Work out the finished part from the listing and answer in its coordinate system (mm). Give positions to 0.01 mm unless a question says otherwise; leave off trailing zeros. One line per question, with ' | ' between items. Start each with the question number.
1. Section A-A (z = 2.75) is taken. Give the number of separate pieces and of enclosed holes in the cut face, plus the area to 3 significant figures.
2. Each of these flat-tipped pins is pushed along its axis until it touches: pin 1 (1 mm diameter, centred on y = 23, z = 3, fed in from +X); pin 2 (2.5 mm diameter, centred on x = 35, y = 0, fed in from +Z); pin 3 (1.8 mm diameter, centred on x = -30.31, y = 17.5, fed in from +Z). Where does it stop, or does it pass through?
3. Find the intervals of material crossed by line 1 (Y direction, x = 30, z = -0.75); line 2 (X direction, y = -18, z = 4); line 3 (Y direction, x = -22.5, z = -2), in increasing order.
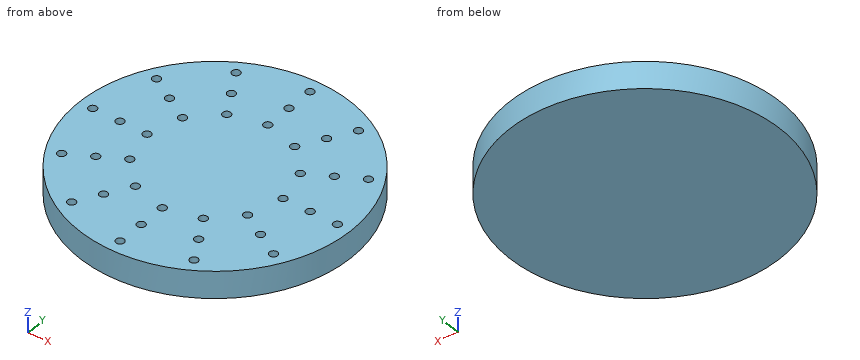
Autodesk Fusion 360 part; units mm, degrees
sketch "base plate" plane through (0, 0, 0) normal (0, 0, 1) x (1, 0, 0)
  circle A0 centre (0, 0) radius 50
  dimension "d1" = 100
extrude "Extrude1" add sketch "base plate" along normal mid plane 10
sketch "tube holes outer layer" plane through (0, 0, 5) normal (0, 0, 1) x (-1, 0, 0)
  circle A0 centre (0, 0) radius 50
  circle A1 centre (45, 0) radius 1.5
  point P0 (-45, 0)
  point P1 (-38.9711, -22.5)
  point P2 (-22.5, -38.9711)
  point P3 (0, -45)
  point P4 (22.5, -38.9711)
  point P5 (38.9711, -22.5)
  point P6 (38.9711, 22.5)
  point P7 (22.5, 38.9711)
  point P8 (0, 45)
  point P9 (-22.5, 38.9711)
  point P10 (-38.9711, 22.5)
  dimension "d4" = 3
  dimension "d6" = 360
hole "Hole1" at (0, 45, 5) at (22.5, 38.9711, 5) at (38.9711, 22.5, 5) at (45, 0, 5) at (38.9711, -22.5, 5) at (22.5, -38.9711, 5) at (0, -45, 5) at (-22.5, -38.9711, 5) at (-38.9711, -22.5, 5) at (-45, 0, 5) at (-38.9711, 22.5, 5) at (-22.5, 38.9711, 5) direction (0, 0, -1) diameter 3 depth 9 tip angle 118
sketch "tube holes layer 2" plane through (0, 0, 5) normal (0, 0, 1) x (-1, 0, 0)
  circle A0 centre (38.9711, -22.5) radius 1.5
  circle A1 centre (38.9711, 22.5) radius 1.5
  circle A2 centre (0, 45) radius 1.5
  circle A3 centre (-38.9711, 22.5) radius 1.5
  circle A4 centre (-38.9711, -22.5) radius 1.5
  circle A5 centre (0, -45) radius 1.5
  circle A6 centre (-22.5, -38.9711) radius 1.5
  circle A7 centre (-45, 0) radius 1.5
  circle A8 centre (-22.5, 38.9711) radius 1.5
  circle A9 centre (22.5, 38.9711) radius 1.5
  circle A10 centre (45, 0) radius 1.5
  circle A11 centre (22.5, -38.9711) radius 1.5
  circle A12 centre (0, 0) radius 50
  line L0 (0, 0) -> (0, -45) construction
  circle A13 centre (0, -35) radius 1.5
  circle A14 centre (0, 35) radius 1.5
  circle A15 centre (-17.5, 30.3109) radius 1.5
  circle A16 centre (-30.3109, 17.5) radius 1.5
  circle A17 centre (-35, 0) radius 1.5
  circle A18 centre (-30.3109, -17.5) radius 1.5
  circle A19 centre (-17.5, -30.3109) radius 1.5
  circle A20 centre (17.5, -30.3109) radius 1.5
  circle A21 centre (30.3109, -17.5) radius 1.5
  circle A22 centre (35, 0) radius 1.5
  circle A23 centre (30.3109, 17.5) radius 1.5
  circle A24 centre (17.5, 30.3109) radius 1.5
  dimension "d10" = 3
  dimension "d12" = 360
hole "Hole2" at (-17.5, 30.3109, 5) at (0, 35, 5) at (17.5, 30.3109, 5) at (30.3109, 17.5, 5) at (35, 0, 5) at (30.3109, -17.5, 5) at (17.5, -30.3109, 5) at (0, -35, 5) at (-17.5, -30.3109, 5) at (-30.3109, -17.5, 5) at (-35, 0, 5) at (-30.3109, 17.5, 5) direction (0, 0, -1) diameter 3 depth 9 tip angle 118
sketch "tube holes layer 3" plane through (0, 0, 5) normal (0, 0, 1) x (-1, 0, 0)
  circle A0 centre (35, 0) radius 1.5
  circle A1 centre (17.5, 30.3109) radius 1.5
  circle A2 centre (-17.5, 30.3109) radius 1.5
  circle A3 centre (-35, 0) radius 1.5
  circle A4 centre (-17.5, -30.3109) radius 1.5
  circle A5 centre (17.5, -30.3109) radius 1.5
  circle A6 centre (0, -35) radius 1.5
  circle A7 centre (-30.3109, -17.5) radius 1.5
  circle A8 centre (-30.3109, 17.5) radius 1.5
  circle A9 centre (0, 35) radius 1.5
  circle A10 centre (30.3109, 17.5) radius 1.5
  circle A11 centre (30.3109, -17.5) radius 1.5
  circle A12 centre (38.9711, -22.5) radius 1.5
  circle A13 centre (38.9711, 22.5) radius 1.5
  circle A14 centre (0, 45) radius 1.5
  circle A15 centre (-38.9711, 22.5) radius 1.5
  circle A16 centre (-38.9711, -22.5) radius 1.5
  circle A17 centre (0, -45) radius 1.5
  circle A18 centre (-22.5, -38.9711) radius 1.5
  circle A19 centre (-45, 0) radius 1.5
  circle A20 centre (-22.5, 38.9711) radius 1.5
  circle A21 centre (22.5, 38.9711) radius 1.5
  circle A22 centre (45, 0) radius 1.5
  circle A23 centre (22.5, -38.9711) radius 1.5
  circle A24 centre (0, 0) radius 50
  circle A25 centre (0, -25) radius 1.5
  point P0 (0, 25)
  point P1 (-12.5, 21.6506)
  point P2 (-21.6506, 12.5)
  point P3 (-25, 0)
  point P4 (-21.6506, -12.5)
  point P5 (-12.5, -21.6506)
  point P6 (12.5, -21.6506)
  point P7 (21.6506, -12.5)
  point P8 (25, 0)
  point P9 (21.6506, 12.5)
  point P10 (12.5, 21.6506)
  dimension "d16" = 3
  dimension "d18" = 360
hole "Hole3" at (0, 25, 5) at (12.5, 21.6506, 5) at (21.6506, 12.5, 5) at (25, 0, 5) at (21.6506, -12.5, 5) at (12.5, -21.6506, 5) at (0, -25, 5) at (-12.5, -21.6506, 5) at (-21.6506, -12.5, 5) at (-25, 0, 5) at (-21.6506, 12.5, 5) at (-12.5, 21.6506, 5) direction (0, 0, -1) diameter 3 depth 9 tip angle 118
Conclusion:
1) separate pieces: 1 | enclosed holes: 36 | area: 7,600 mm²
2) pin 1: x = 44.65 | pin 2: z = -4.15 | pin 3: z = -4.36
3) line 1: -40 to -18.97, -16.03 to 16.03, 18.97 to 40 | line 2: -46.65 to -31.73, -28.9 to 28.9, 31.73 to 46.65 | line 3: -44.65 to -40.47, -37.47 to -13.74, -11.26 to 11.26, 13.74 to 37.47, 40.47 to 44.65
